from build123d import *

# Parameters (mm, degrees)
EXTRUDE_3_DEPTH     = 500
SKETCH_2_R          = 2.2
SKETCH_2_W          = 8.2
SKETCH_2_H          = 14
CUT_EXTRUDE_1_DEPTH = 8.148528137


with BuildPart() as part:
    # Эскиз1 → Вытянуть-Тонкостенный3 (new body)
    with BuildSketch(Plane(origin=(0, 0, 0), x_dir=(0, 0, -1), z_dir=(1, 0, 0))):
        with BuildLine():
            Line((6.3, 11.5), (5.501920783, 10.701920783))
            Line((5.501920783, 10.701920783), (4.371381229, 10.701920783))
            Line((4.371381229, 10.701920783), (3.573302011, 11.5))
            Line((3.573302011, 11.5), (1, 11.5))
            ThreePointArc((1, 11.5), (0.292893219, 11.207106781), (0, 10.5))
            Line((0, 10.5), (0, -10.5))
            ThreePointArc((0, -10.5), (0.292893219, -11.207106781), (1, -11.5))
            Line((1, -11.5), (3.573302011, -11.5))
            Line((3.573302011, -11.5), (4.371381229, -10.701920783))
            Line((4.371381229, -10.701920783), (5.501920783, -10.701920783))
            Line((5.501920783, -10.701920783), (6.3, -11.5))
            Line((6.3, -11.5), (7.148528137, -10.651471863))
            Line((7.148528137, -10.651471863), (5.998977057, -9.501920783))
            Line((5.998977057, -9.501920783), (3.874324954, -9.501920783))
            Line((3.874324954, -9.501920783), (3.076245737, -10.3))
            Line((3.076245737, -10.3), (1.2, -10.3))
            Line((1.2, -10.3), (1.2, 10.3))
            Line((1.2, 10.3), (3.076245737, 10.3))
            Line((3.076245737, 10.3), (3.874324954, 9.501920783))
            Line((3.874324954, 9.501920783), (5.998977057, 9.501920783))
            Line((5.998977057, 9.501920783), (7.148528137, 10.651471863))
            Line((7.148528137, 10.651471863), (6.3, 11.5))
        make_face()
    extrude(amount=EXTRUDE_3_DEPTH)

    # Эскиз2 → Вырез-Вытянуть1 (cut, through all)
    with BuildSketch(Plane.XY):
        with Locations((449.6, 0)):
            Circle(SKETCH_2_R)
        with Locations((226.6, 0)):
            Circle(SKETCH_2_R)
        with Locations((33.6, 0)):
            Circle(SKETCH_2_R)
        with Locations((495.9, 0)):
            Rectangle(SKETCH_2_W, SKETCH_2_H)
        with BuildLine():
            Line((472, 2.2), (477, 2.2))
            ThreePointArc((477, 2.2), (479.2, 0), (477, -2.2))
            Line((477, -2.2), (472, -2.2))
            ThreePointArc((472, -2.2), (469.8, 0), (472, 2.2))
        make_face()
        with BuildLine():
            Line((456.4, 1.779598361), (456.4, -2.5))
            ThreePointArc((456.4, -2.5), (458.6, -4.7), (460.8, -2.5))
            Line((460.8, -2.5), (460.8, 1.779598361))
            ThreePointArc((460.8, 1.779598361), (458.6, 3.979598361), (456.4, 1.779598361))
        make_face()
        with BuildLine():
            Line((233.4, 1.779598361), (233.4, -2.5))
            ThreePointArc((233.4, -2.5), (235.6, -4.7), (237.8, -2.5))
            Line((237.8, -2.5), (237.8, 1.779598361))
            ThreePointArc((237.8, 1.779598361), (235.6, 3.979598361), (233.4, 1.779598361))
        make_face()
        with BuildLine():
            Line((249, -2.2), (254, -2.2))
            ThreePointArc((254, -2.2), (256.2, 0), (254, 2.2))
            Line((254, 2.2), (249, 2.2))
            ThreePointArc((249, 2.2), (246.8, 0), (249, -2.2))
        make_face()
        with BuildLine():
            Line((44.8, -2.5), (44.8, 1.779598361))
            ThreePointArc((44.8, 1.779598361), (42.6, 3.979598361), (40.4, 1.779598361))
            Line((40.4, 1.779598361), (40.4, -2.5))
            ThreePointArc((40.4, -2.5), (42.6, -4.7), (44.8, -2.5))
        make_face()
        with BuildLine():
            Line((56, 2.2), (61, 2.2))
            ThreePointArc((61, 2.2), (63.2, 0), (61, -2.2))
            Line((61, -2.2), (56, -2.2))
            ThreePointArc((56, -2.2), (53.8, 0), (56, 2.2))
        make_face()
    extrude(amount=-CUT_EXTRUDE_1_DEPTH, mode=Mode.SUBTRACT)


solid = part.part
Can you work these out from the model? Positions are in its coordinate system, mm. Coordinates: 2 decimals unless noted, no trailing zeros. Loops run counter-clockwise (first coordinate to the right, second up) from the corner with the lowest first, then second, coordinate; pieces in that order, holes last. Notation, with made-up numbers: (82.5, 53) - (133.5, 53) arc R23 ccw to (133.5, 78) - close; hole circle Ø8 at (16.25, 18). An arc over 180 degrees is marked (long way). Answer as a JSON object with one key per item and string values. Group by question number.
Item 1: If I drill on L1, parallel to Y at x = 249, z = -5.5; L2, parallel to Y at x = 72, z = -2.5; L3, parallel to X at y = 3.25, z = -0.25, over which ranges is the centre line in solid material (lowest first)? Write a range as from..to.
Item 2: If we mould it in two halves opening along Y, with no side actions, what happens to faces 1 (the face through (246, 0, -1.2)), 2 (the face through (246, 0, 0))? For each: released by +Y, released by -Y, zero draft, split by the parting line, or undercut.
Item 3: If we section it at A-A (x = 365): List the corners of the cut face in (y, z) for me.
Item 4: For pin 1 (1.7 mm diameter, centred on x = 150, z = -5, fed in from +Y); pin 2 (1.3 mm diameter, centred on y = -1, z = -0.5, fed in from +X); pin 3 (6 mm diameter, centred on x = 139, y = -1, fed in from -Z); pin 4 (2.5 mm diameter, centred on x = 226.6, y = 0, fed in from +Z), each with a flat end and sliding along its axis, tell me the tip position at first contact or that it passes through.
Returned:
{
 "1": {"L1": "y = -10.7..-9.5, 9.5..10.7", "L2": "y = -11.5..-10.3, 10.3..11.5", "L3": "x = 0..40.96, 44.24..233.96, 237.24..456.96, 460.24..491.8"},
 "2": {"face 1": "undercut", "face 2": "zero draft"},
 "3": {"outline": "(-11.5, -6.3) - (-10.65, -7.15) - (-9.5, -6) - (-9.5, -3.87) - (-10.3, -3.08) - (-10.3, -1.2) - (10.3, -1.2) - (10.3, -3.08) - (9.5, -3.87) - (9.5, -6) - (10.65, -7.15) - (11.5, -6.3) - (10.7, -5.5) - (10.7, -4.37) - (11.5, -3.57) - (11.5, -1) arc R1 ccw to (10.5, 0) - (-10.5, 0) arc R1 ccw to (-11.5, -1) - (-11.5, -3.57) - (-10.7, -4.37) - (-10.7, -5.5) - close"},
 "4": {"pin 1": "stops at y = 11.05", "pin 2": "stops at x = 491.8", "pin 3": "stops at z = -1.2", "pin 4": "passes through"}
}
